Can you work these out from the model? Positions are in its coordinate system, mm. A direction names the side the tool comes from. Give positions to 0.01 mm unless a question says otherwise; leave off trailing zeros. Loops run counter-clockwise (first coordinate to the right, second up) from the corner with the lowest first, then second, coordinate; pieces in that order, holes last. Notation, with made-up numbers: M 11,-19 L 49,-19 A6 cw 49,-9 Z; hole C 51.25,-26.75 d9. An arc over 180 degrees is marked long. Use CSV: the item, a comma, the result in double quotes.
from build123d import *

# Parameters (mm, degrees)
F2_W     = 508
F2_H     = 381
F2_R     = 15.24
F3_DEPTH = 25.4
F4_W     = 25.4
F4_H     = 25.4
F5_DEPTH = 297.18
F7_DEPTH = 2.54


with BuildPart() as f3:
    # F2 (on face) → F3 (new body)
    with BuildSketch(Plane.XY):
        with Locations((-12.433536, 36.703804)):
            Rectangle(F2_W, F2_H)
        with Locations((-225.793536, -62.356196)):
            Circle(F2_R, mode=Mode.SUBTRACT)
    extrude(amount=F3_DEPTH)

    # F4 (on face) → F5 (join)
    with BuildSketch(Plane.XY):
        with Locations((-253.733536, -141.096196)):
            Rectangle(F4_W, F4_H)
        with Locations((228.866464, 214.503804)):
            Rectangle(F4_W, F4_H)
        with Locations((228.866464, -141.096196)):
            Rectangle(F4_W, F4_H)
        with Locations((-253.733536, 214.503804)):
            Rectangle(F4_W, F4_H)
    extrude(amount=-F5_DEPTH)

    # F6 (on face) → F7 (join)
    with BuildSketch(Plane.XY):
        Polygon((-78.894847, -45.385379), (-82.638033, -41.965879), (-128.514952, -65.7849), (-126.283888, -70.082069), align=None)
    extrude(amount=-F7_DEPTH)


solid = f3.part
Q1. Please list where this line runs through material, in increasing order: L1, parallel to Z at x = 77, y = 114.5. Write a range as from..to.
Model answer:
L1,"0..25.4"
Q2. For faces 1 (the flat face through (-254, -128.396, -147)), 2 (the flat face through (229, -141, -297.18)), 3 (the flat face through (-102.921, -57.907, -1.252)), 4 (the flat face through (-241.034, -141, -147)), which set-ups out of +Z, -Z, +X, -X, +Y, -Y let a thin tool reach every point of the face, with its end or its side?
Model answer:
face 1,"-Z, +X, -X"
face 2,"-Z, +X, -X, +Y, -Y"
face 3,"-Z, +X, -Y"
face 4,"-Z, +Y, -Y"
Q3. I want a section at C-C, the plane y = 167.5. Please give me the cut outline in (x, z), then the cut area to 3 significant figures.
Model answer:
outline,"M -266.43,0 L 241.57,0 L 241.57,25.4 L -266.43,25.4 Z"
area,"12,900 mm2"
Q4. I want a section at A-A, the plane z = -40.5. Please give me the cut outline in (x, y).
Model answer:
outline,"M -266.43,-153.8 L -241.03,-153.8 L -241.03,-128.4 L -266.43,-128.4 Z; M -266.43,201.8 L -241.03,201.8 L -241.03,227.2 L -266.43,227.2 Z; M 216.17,-153.8 L 241.57,-153.8 L 241.57,-128.4 L 216.17,-128.4 Z; M 216.17,201.8 L 241.57,201.8 L 241.57,227.2 L 216.17,227.2 Z"
Q5. If we mould it in two halves opening along Y, with no side actions, what happens to faces 5 (the flat face through (-32, -153.796, 8)), 6 (the flat face through (-105.26, -53.71, -1.25)), 7 (the flat face through (-266.434, 8, 8)), 8 (the cylindrical face through (-241.02, -61.69, 12.52))? For each: released by +Y, released by -Y, zero draft, split by the parting line, or undercut.
Model answer:
face 5,"released by -Y"
face 6,"released by +Y"
face 7,"zero draft"
face 8,"undercut"
Q6. I want a section at B-B, the plane x = 208. Please give me the cut outline in (y, z).
Model answer:
outline,"M -153.8,0 L 227.2,0 L 227.2,25.4 L -153.8,25.4 Z"
Q7. I'm going to push flat-ended pins straight in: P1, Ø2, axis at x = 97, y = -36, coming from the -Z side; P2, Ø8.5, axis at x = -95.5, y = -53.5, coming from the -Z side. Where does each tip first touch, or does it pass through?
Model answer:
P1,"z = 0"
P2,"z = -2.54"
